Verification items for this drawing (mm, ordinates from the low corner). Round coordinates to 2 decimals unless told otherwise and drop trailing zeros. Loops run counter-clockwise (first coordinate to the right, second up) from the corner with the lowest first, then second, coordinate; pieces in that order, holes last. Notation, with made-up numbers: M 41.5,-22 L 96.5,-22 A15 cw 96.5,6 Z; hole C 1.25,-7.5 d3. An arc over 180 degrees is marked long. Write item = value, one per line. Start each with the question number.
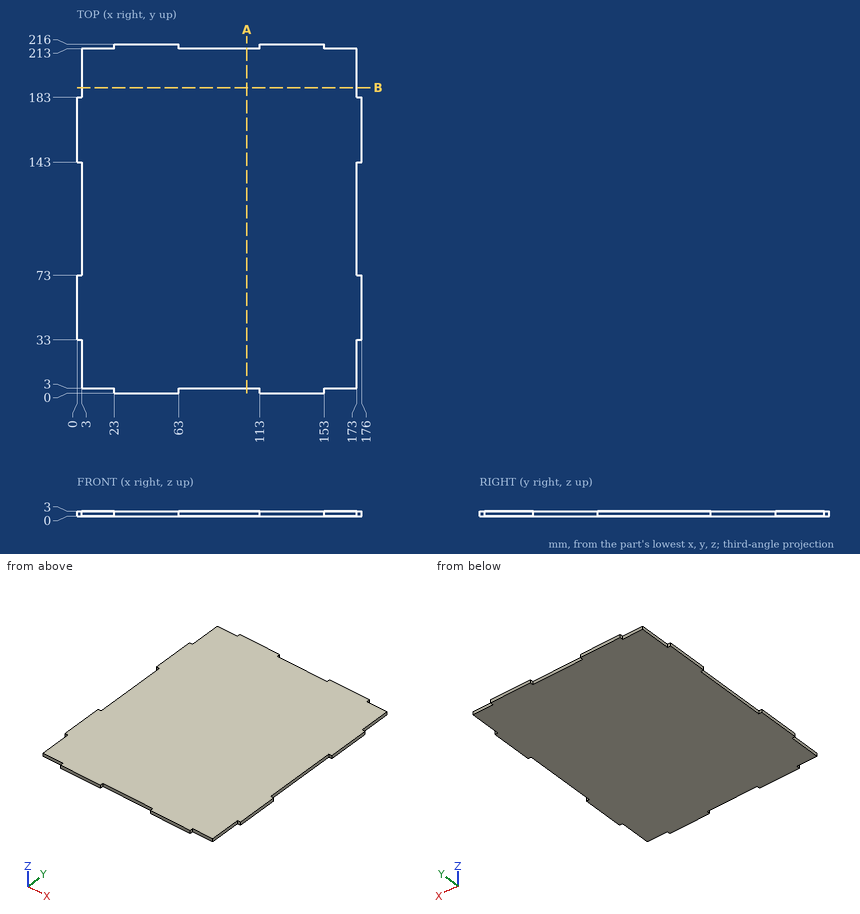
1. Section check A-A, the plane x = 105. Enter the section's corners in (y, z).
2. Thickness scan on line 1 (X direction, y = 97.5, z = 2.5); line 2 (Y direction, x = 21, z = 1.7). Record the ranges inside material, lowest first.
3. Gauge pin test, flat ends, axial feed: P1, Ø0.9, axis at x = 174.5, z = 2, coming from the +Y side; P2, Ø1.5, axis at x = 16.5, z = 1.5, coming from the -Y side; P3, Ø1.5, axis at y = 214, z = 2, coming from the +X side. Record the tip position at first contact, or that the pin passes through.
4. Section check B-B, the plane y = 189. Enter the section's corners in (x, z).
Computed values:
q1.outline = M 3,0 L 213,0 L 213,3 L 3,3 Z
q2.line_1 = 3 to 173
q2.line_2 = 3 to 213
q3.P1 = 183
q3.P2 = 3
q3.P3 = 153
q4.outline = M 3,0 L 173,0 L 173,3 L 3,3 Z
